from build123d import *

# Parameters (mm, degrees)
SKETCH1_R               = 2.5
BOSS_EXTRUDE1_DEPTH     = 5
FILLET1_R               = 10
SKETCH2_W               = 40
SKETCH2_H               = 5
BOSS_EXTRUDE2_DEPTH     = 40
SKETCH3_R               = 2.5
CUT_EXTRUDE1_DEPTH      = 106.814430788
FILLET3_R               = 10
SKETCH4_W               = 2
SKETCH4_H               = 7
BOSS_EXTRUDE3_DEPTH     = 8
CUT_EXTRUDE2_DEPTH      = 109.89140498
CUT_EXTRUDE2_DEPTH_BACK = 109.89140498
SKETCH5_W               = 6
SKETCH5_H               = 5


with BuildPart() as part:
    # Sketch1 → Boss-Extrude1 (new body)
    with BuildSketch(Plane.XY):
        Polygon((0, 90), (80, 90), (53.46739399, 30), (26.53260601, 30), align=None)
        with Locations((15, 80)):
            Circle(SKETCH1_R, mode=Mode.SUBTRACT)
        with Locations((65, 80)):
            Circle(SKETCH1_R, mode=Mode.SUBTRACT)
        with Locations((40, 35)):
            Circle(SKETCH1_R, mode=Mode.SUBTRACT)
        with Locations((40, 65)):
            Circle(SKETCH1_R, mode=Mode.SUBTRACT)
    extrude(amount=BOSS_EXTRUDE1_DEPTH)

    # Fillet1
    fillet1_edges = [part.edges().sort_by_distance(p)[0] for p in [
        (0, 90, 2.5),
        (80, 90, 2.5),
        (53.46739399, 30, 2.5),
        (26.53260601, 30, 2.5),
    ]]
    fillet(fillet1_edges, radius=FILLET1_R)

    # Sketch2 → Boss-Extrude2 (add)
    with BuildSketch(Plane.XY.offset(5)):
        with Locations((40, 87.5)):
            Rectangle(SKETCH2_W, SKETCH2_H)
    extrude(amount=BOSS_EXTRUDE2_DEPTH)

    # Sketch3 → Cut-Extrude1 (cut, through all)
    with BuildSketch(Plane(origin=(0, 90, 0), x_dir=(1, 0, 0), z_dir=(0, 1, 0))):
        with Locations(Location((40, -15, 0), (0, 0, 180))):
            Circle(SKETCH3_R)
        with Locations(Location((40, -35, 0), (0, 0, 180))):
            Circle(SKETCH3_R)
    extrude(amount=-CUT_EXTRUDE1_DEPTH, mode=Mode.SUBTRACT)

    # Fillet3
    fillet3_edges = [part.edges().sort_by_distance(p)[0] for p in [
        (60, 87.5, 5),
        (20, 87.5, 5),
    ]]
    fillet(fillet3_edges, radius=FILLET3_R)

    # Sketch4 → Boss-Extrude3 (add)
    with BuildSketch(Plane(origin=(0, 0, 0), x_dir=(-1, 0, 0), z_dir=(0, 0, -1))):
        with Locations((-34.022413797, 33.5)):
            Rectangle(SKETCH4_W, SKETCH4_H)
        with Locations((-45.977586203, 33.5)):
            Rectangle(SKETCH4_W, SKETCH4_H)
    extrude(amount=BOSS_EXTRUDE3_DEPTH)

    # Sketch5 → Cut-Extrude2 (cut, two sides: drawn at the far end of the back side and taken through both)
    with BuildSketch(Plane(origin=(46.977586203, 0, 0), x_dir=(0, 0, -1), z_dir=(1, 0, 0)).offset(-CUT_EXTRUDE2_DEPTH_BACK)):
        with Locations((4.124970421, 33.5)):
            Rectangle(SKETCH5_W, SKETCH5_H)
    extrude(amount=CUT_EXTRUDE2_DEPTH + CUT_EXTRUDE2_DEPTH_BACK, mode=Mode.SUBTRACT)


solid = part.part
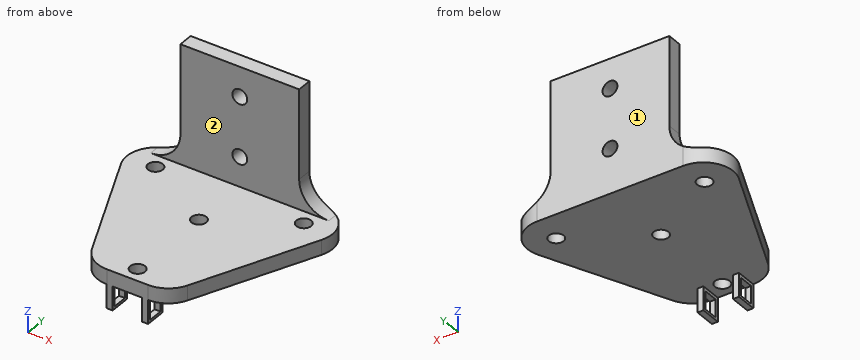
Here's how the part is built. I have some questions about the finished solid (model axes, mm). Face numbers are marked on the shaded views. A direction names the side the tool comes from. Round coordinates to 2 decimals unless told otherwise and drop trailing zeros. Order: outer loops, then holes, each group sorted by start corner. A loop starts at its lowest first (then second) coordinate and runs counter-clockwise, first axis right, second up. Notation, with made-up numbers: M -20.5,-4 L -16.5,-4 A29 cw -16.5,31 Z; hole C -6,-11.5 d2. An arc over 180 degrees is marked long. One line per question, with ' | ' between items.
1) Imagine slicing it at A-A, the plane x = 40. Write out the boundary of the cut face in (y, z).
Checked values:
outline: M 30,0 L 32.5,0 L 32.5,5 L 30,5 Z; M 37.5,0 L 62.5,0 L 62.5,5 L 37.5,5 Z; M 67.5,0 L 90,0 L 90,12.5 L 85,12.5 L 85,5 L 67.5,5 Z; M 85,17.5 L 90,17.5 L 90,32.5 L 85,32.5 Z; M 85,37.5 L 90,37.5 L 90,45 L 85,45 Z
2) Imagine slicing it at C-C, the plane y = 80. Write out the boundary of the cut face in (x, z).
Checked values:
outline: M 5.36,0 L 12.5,0 L 12.5,5 L 5.36,5 Z; M 17.5,0 L 62.5,0 L 62.5,5 L 17.5,5 Z; M 67.5,0 L 74.64,0 L 74.64,5 L 67.5,5 Z
3) Imagine slicing it at B-B, the plane z = 35. Write out the boundary of the cut face in (x, y).
Checked values:
outline: M 20,85 L 37.5,85 L 37.5,90 L 20,90 Z; M 42.5,85 L 60,85 L 60,90 L 42.5,90 Z
4) I'm going to push flat-ended pins straight in: pin 1 Ø4 at (x, z) = (38, 17) entering from -Y; pin 2 Ø2 at (x, y) = (33.5, 34.5) entering from +Z; pin 3 Ø5 at (y, z) = (74.5, 7) entering from -X. Where does each tip first touch, or does it pass through?
Checked values:
pin 1: stops at y = 85 | pin 2: stops at z = 5 | pin 3: stops at x = 6.19
5) I need wall thicknesses on line 1 (Z direction, x = 40, y = 87.2); line 2 (Y direction, x = 65, z = 3); line 3 (Y direction, x = 40, z = 1). Which ranges of each line are inside material? Lowest first, please.
Checked values:
line 1: z = 0 to 12.5, 17.5 to 32.5, 37.5 to 45 | line 2: y = 56.08 to 77.5, 82.5 to 89.99 | line 3: y = 30 to 32.5, 37.5 to 62.5, 67.5 to 90
6) On a 3-axis mill with a long thin cutter (end or side, diameter ignored), from which of +Z, -Z, +X, -X, +Y, -Y can I reach the whole of each face in a straight line? I mean the marked faces 1 and 2. Say none if no direction works.
Checked values:
face 1: +Z, -Z, +X, -X, +Y | face 2: +Z, +X, -X, -Y
7) Imagine slicing it at D-D, the plane z = -3. Write out the boundary of the cut face in (x, y), plus the area to 3 significant figures.
Checked values:
outline: M 33.02,30 L 35.02,30 L 35.02,31 L 33.02,31 Z; M 33.02,36 L 35.02,36 L 35.02,37 L 33.02,37 Z; M 44.98,30 L 46.98,30 L 46.98,31 L 44.98,31 Z; M 44.98,36 L 46.98,36 L 46.98,37 L 44.98,37 Z | area: 8.00 mm²
